Read the model definition and answer for the solid it produces. Units are mm, in the model's axes. Coordinates: 2 decimals unless noted, no trailing zeros. Write each loop counter-clockwise with the first axis right and the second up, starting at its lowest first coordinate (ties: lowest second). Pieces come first, ordered by that corner, then holes.
1) The part is cut by section A-A (x = 0). Determine the outline of the cut face in (y, z) (1 decimal).
2) Find the intervals of material crossed by line 1 (X direction, y = 0, z = -4) (1 decimal); line 2 (Y direction, x = -1, z = 0.25) (3 decimals), in increasing order.
3) The part is cut by section C-C (z = -2.25). Determine the outline of the cut face in (x, y) (1 decimal), then the cut area to 3 significant figures.
4) This flat-tipped pin is pushed along its axis until it touches: pin 1 Ø4 at (x, y) = (1, -1) entering from -Z. Where does it stop, or does it pass through?
from build123d import *

# Parameters (mm, degrees)
F0_W     = 19.05
F0_H     = 19.05
F0_R     = 4.7625
F1_DEPTH = 9.525
F2_ANGLE = 90


with BuildPart() as f1:
    # F0 (on Front) → F1 (new body, symmetric)
    with BuildSketch(Plane.XZ):
        Rectangle(F0_W, F0_H)
        Circle(F0_R, mode=Mode.SUBTRACT)
    extrude(amount=F1_DEPTH, both=True)


with BuildPart() as f1_1:
    # F2: moved
    add(f1.part.rotate(Axis((4.7625, 0, 0), (1, 0, 0)), F2_ANGLE))


solid = f1_1.part
Reported:
1. outline: (-9.5, -9.5) - (-4.8, -9.5) - (-4.8, 9.5) - (-9.5, 9.5) - close; (4.8, -9.5) - (9.5, -9.5) - (9.5, 9.5) - (4.8, 9.5) - close
2. line 1: x = -9.5 to -4.8, 4.8 to 9.5
2. line 2: y = -9.525 to -4.656, 4.656 to 9.525
3. outline: (-9.5, -9.5) - (9.5, -9.5) - (9.5, 9.5) - (-9.5, 9.5) - close; hole circle Ø9.5 at (0, 0)
3. area: 292 mm2
4. pin 1: passes through
